For this review, use the dimensioned drawing (mm, ordinates from the lowest corner) and the shaded views. A direction names the side the tool comes from. Coordinates: 2 decimals unless noted, no trailing zeros. Write each loop counter-clockwise with the first axis right and the second up, starting at its lowest first coordinate (ties: lowest second). Pieces come first, ordered by that corner, then holes. Notation, with made-up numbers: (43, 60.5) - (80, 60.5) arc R21 cw to (80, 99.5) - close; hole circle Ø8 at (21.5, 41.25). An arc over 180 degrees is marked (long way). One line per item, written item: value.
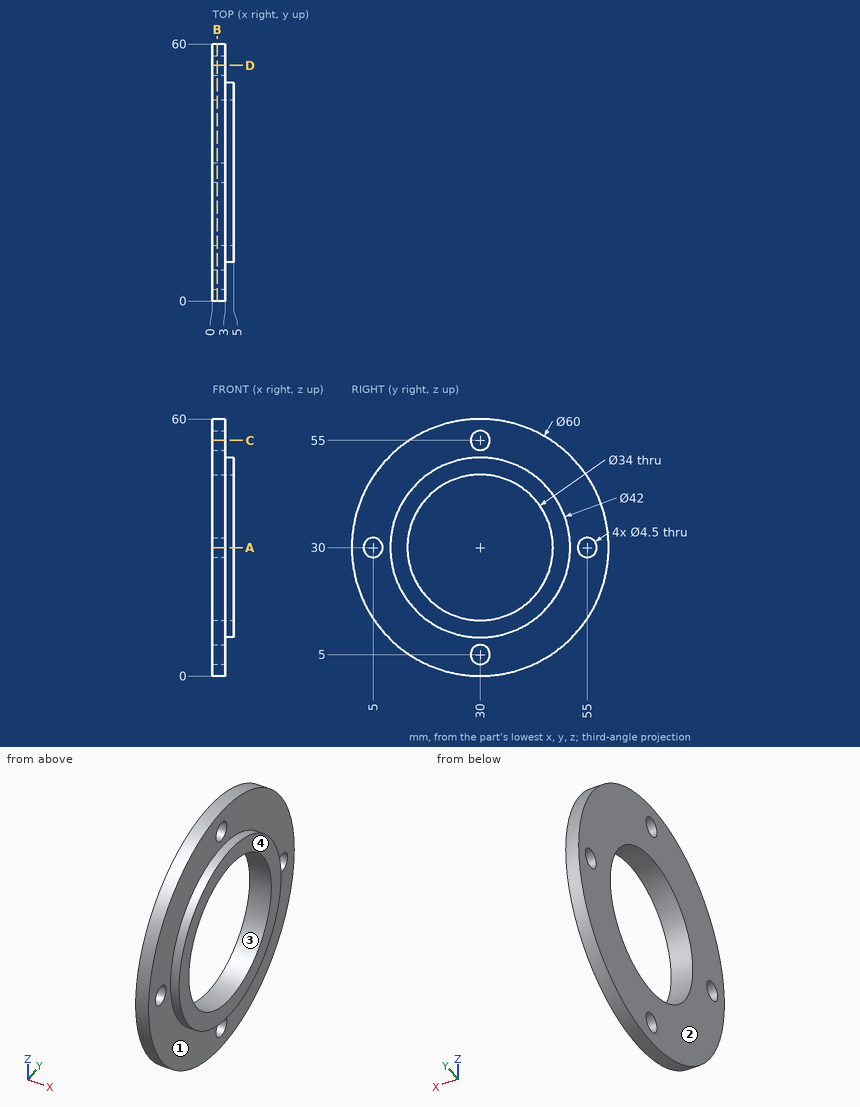
1. Insertion check: pin 1 Ø3 at (x, z) = (0.5, 52) entering from +Y; pin 2 Ø2 at (y, z) = (7, 32) entering from +X; pin 3 Ø3 at (x, y) = (2.5, 14) entering from -Z. Each pin has a flat end and moves straight along its axis. Give the tip position at first contact, or say it passes through.
Answer block:
pin 1: stops at y = 51.9
pin 2: stops at x = 3
pin 3: stops at z = 3.74
2. Mouldability with a two-part tool opening along Y and no side actions: class the marked faces 3 and 4 as released by +Y, released by -Y, zero draft, split by the parting line, or undercut.
Answer block:
face 3: undercut
face 4: zero draft
3. Consider section C-C, the plane z = 55. Write out the cut boundary in (x, y).
Answer block:
outline: (0, 13.42) - (3, 13.42) - (3, 27.75) - (0, 27.75) - close; (0, 32.25) - (3, 32.25) - (3, 46.58) - (0, 46.58) - close
4. Wall thickness on line 1 along Z through (x, y) = (0.6, 30); line 2 along Y through (x, z) = (1.8, 29.5); line 3 along Y through (x, z) = (1, 28.5): over which ranges is each line inside the solid? List them lowest first.
Answer block:
line 1: z = 0 to 2.75, 7.25 to 13, 47 to 52.75, 57.25 to 60
line 2: y = 0 to 2.81, 7.19 to 13.01, 46.99 to 52.81, 57.19 to 60
line 3: y = 0.04 to 3.32, 6.68 to 13.07, 46.93 to 53.32, 56.68 to 59.96
5. Consider section B-B, the plane x = 1.15. Write out the cut boundary in (y, z).
Answer block:
outline: circle Ø60 at (30, 30); hole circle Ø4.5 at (5, 30); hole circle Ø34 at (30, 30); hole circle Ø4.5 at (30, 5); hole circle Ø4.5 at (30, 55); hole circle Ø4.5 at (55, 30)
6. For the marked faces 1 and 2, list the 3-axis set-ups (+Z, -Z, +X, -X, +Y, -Y) from which the entire face can be reached by the end or side of a thin tool; tool diameter is ignored.
Answer block:
face 1: +X
face 2: +Z, -Z, -X, +Y, -Y
7. Consider section A-A, the plane z = 30. Write out the cut boundary in (x, y).
Answer block:
outline: (0, 0) - (3, 0) - (3, 2.75) - (0, 2.75) - close; (0, 7.25) - (3, 7.25) - (3, 9) - (5, 9) - (5, 13) - (0, 13) - close; (0, 47) - (5, 47) - (5, 51) - (3, 51) - (3, 52.75) - (0, 52.75) - close; (0, 57.25) - (3, 57.25) - (3, 60) - (0, 60) - close
